from build123d import *

# Parameters (mm, degrees)
FILLET1_R     = 1.5
CHAMFER1_SIZE = 0.5


with BuildPart() as part:
    # Sketch1 → Revolve1 (revolve)
    with BuildSketch(Plane.XY, mode=Mode.PRIVATE) as revolve1_sk:
        with BuildLine():
            Line((-11.000013874, -2.81e-07), (-1, -2.81e-07))
            Line((-1, -2.81e-07), (-1, -5.000000281))
            Line((-1, -5.000000281), (0, -5.000000281))
            Line((0, -5.000000281), (0, 5.06243))
            Line((0, 5.06243), (-1.5, 5.06243))
            ThreePointArc((-1.5, 5.06243), (-6.215053401, 4.581844183), (-10.565043576, 2.700281861))
            ThreePointArc((-10.565043576, 2.700281861), (-11.252524354, 1.971118503), (-11.499986126, 0.999999718))
            Line((-11.499986126, 0.999999718), (-11.5, 0.499999719))
            ThreePointArc((-11.5, 0.499999719), (-11.353562359, 0.14644717), (-11.000013874, -2.81e-07))
        make_face()
    revolve(revolve1_sk.sketch.rotate(Axis((0, 0, 0), (0, 1, 0)), 270), axis=Axis((0, 0, 0), (0, 1, 0)))

    # Fillet1
    fillet1_edges = [part.edges().sort_by_distance(p)[0] for p in [
        (0, -2.813517580805419e-07, 1.0),
    ]]
    fillet(fillet1_edges, radius=FILLET1_R)

    # Chamfer1
    chamfer1_edges = [part.edges().sort_by_distance(p)[0] for p in [
        (0, -5.000000281, 1),
    ]]
    chamfer(chamfer1_edges, length=CHAMFER1_SIZE)


solid = part.part
For this review, take the finished solid that the model builds, in its own axes (mm). Round coordinates to 2 decimals unless told otherwise and drop trailing zeros. Order: outer loops, then holes, each group sorted by start corner. A loop starts at its lowest first (then second) coordinate and runs counter-clockwise, first axis right, second up. Notation, with made-up numbers: M 47,-13.5 L 74,-13.5 A35 cw 74,24.5 Z; hole C 51,13.5 d9. An arc over 180 degrees is marked long. Write each question's results on one line, items separated by ' | '. Start each with the question number.
1. To check wall thickness, follow L1, parallel to Y at x = 5, z = 6.75; L2, parallel to Y at x = -1.5, z = -7.75; L3, parallel to Z at x = -9, y = 1.5. State the ranges of each line that lie inside material, in increasing order. Write a range as [from, to].
2. Clearance check with flat-ended pins moving along their axes: pin 1 Ø4 at (y, z) = (-1, 6) entering from -X; pin 2 Ø10 at (x, z) = (-7.5, 2) entering from +Y; pin 3 Ø6 at (x, y) = (9, -2) entering from -Z. State where each tip first meets the part, or that it passes through.
3. Draft analysis for pull direction Z (two halves, no side actions). For faces 1 (the face through (0, 5.062, 0)), 2 (the face through (-3.45, 0.75, -10.97)), 3 (the face through (0, -5, 0)), state which applies: pulls with the +Z half, pulls with the -Z half, needs draft (parallel to the pull), parting line crosses it, or undercut.
4. Add section A-A (y = -3). State the section outline as (x, z) points.
Output values:
1) L1: [0, 3.83] | L2: [0, 4.04] | L3: [-7.06, 7.06]
2) pin 1: x = -10.55 | pin 2: y = 5.08 | pin 3: z = -9.03
3) face 1: undercut | face 2: parting line crosses it | face 3: needs draft
4) outline: C 0,0 d2
